```python
from build123d import *

# Parameters (mm, degrees)
BOSS_EXTRUDE1_DEPTH = 17
SKETCH2_W           = 17
SKETCH2_H           = 17
CUT_EXTRUDE1_DEPTH  = 13
SKETCH3_RX          = 4.47
SKETCH3_RY          = 3.075
CUT_EXTRUDE2_DEPTH  = 13
SKETCH5_RX          = 4.47
SKETCH5_RY          = 3.075
CUT_EXTRUDE3_DEPTH  = 13
SKETCH6_W           = 3.5
SKETCH6_H           = 1.5
BOSS_EXTRUDE2_DEPTH = 1
FILLET1_R           = 0.75
SKETCH7_W           = 1.5
SKETCH7_H           = 3.5
BOSS_EXTRUDE3_DEPTH = 1
FILLET2_R           = 0.75


with BuildPart() as part:
    # Sketch1 → Boss-Extrude1 (new body)
    with BuildSketch(Plane.XY):
        Polygon((0, 0), (0, 20), (3.029437252, 20), (20, 3.029437252), (20, 0), align=None)
    extrude(amount=BOSS_EXTRUDE1_DEPTH)

    # Sketch2 → Cut-Extrude1 (cut)
    with BuildSketch(Plane.XY.offset(2)):
        with Locations((11.5, 11.5)):
            Rectangle(SKETCH2_W, SKETCH2_H)
    extrude(amount=CUT_EXTRUDE1_DEPTH, mode=Mode.SUBTRACT)

    # Sketch3 → Cut-Extrude2 (cut)
    with BuildSketch(Plane(origin=(0, 0, 0), x_dir=(1, 0, 0), z_dir=(0, 1, 0))):
        with Locations((10.16, -8.425)):
            Ellipse(SKETCH3_RX, SKETCH3_RY)
    extrude(amount=CUT_EXTRUDE2_DEPTH, mode=Mode.SUBTRACT)

    # Sketch5 → Cut-Extrude3 (cut)
    with BuildSketch(Plane(origin=(0, 0, 0), x_dir=(0, 0, -1), z_dir=(1, 0, 0))):
        with Locations(Location((-8.375, 10.47), (0, 0, 90))):
            Ellipse(SKETCH5_RX, SKETCH5_RY)
    extrude(amount=CUT_EXTRUDE3_DEPTH, mode=Mode.SUBTRACT)

    # Sketch6 → Boss-Extrude2 (add)
    with BuildSketch(Plane(origin=(0, 0, 0), x_dir=(0, 0, -1), z_dir=(1, 0, 0))):
        with Locations((-8.25, 18.25)):
            Rectangle(SKETCH6_W, SKETCH6_H)
        with Locations((-8.25, 2.75)):
            Rectangle(SKETCH6_W, SKETCH6_H)
    extrude(amount=-BOSS_EXTRUDE2_DEPTH)

    # Fillet1
    fillet1_edges = [part.edges().sort_by_distance(p)[0] for p in [
        (-0.5, 2, 6.5),
        (-0.5, 17.5, 6.5),
        (-0.5, 2, 10),
        (-0.5, 3.5, 10),
        (-0.5, 3.5, 6.5),
        (-0.5, 17.5, 10),
        (-0.5, 19, 10),
        (-0.5, 19, 6.5),
    ]]
    fillet(fillet1_edges, radius=FILLET1_R - 0.0001)  # a hair under: the kernel refuses the full size

    # Sketch7 → Boss-Extrude3 (add)
    with BuildSketch(Plane(origin=(0, 0, 0), x_dir=(1, 0, 0), z_dir=(0, 1, 0))):
        with Locations((2.75, -8.25)):
            Rectangle(SKETCH7_W, SKETCH7_H)
        with Locations((18.25, -8.25)):
            Rectangle(SKETCH7_W, SKETCH7_H)
    extrude(amount=-BOSS_EXTRUDE3_DEPTH)

    # Fillet2
    fillet2_edges = [part.edges().sort_by_distance(p)[0] for p in [
        (3.5, -0.5, 6.5),
        (2, -0.5, 6.5),
        (2, -0.5, 10),
        (3.5, -0.5, 10),
        (17.5, -0.5, 10),
        (19, -0.5, 10),
        (17.5, -0.5, 6.5),
        (19, -0.5, 6.5),
    ]]
    fillet(fillet2_edges, radius=FILLET2_R - 0.0001)  # a hair under: the kernel refuses the full size


solid = part.part
```
Geometry: final body of the model. Coordinates: model frame, mm. A direction names the side the tool comes from. Round coordinates to 2 decimals unless told otherwise and drop trailing zeros. Write each loop counter-clockwise with the first axis right and the second up, starting at its lowest first coordinate (ties: lowest second). Pieces come first, ordered by that corner, then holes. Notation, with made-up numbers: (-39, -22) -> (-30, -22) arc R11 ccw to (-30, -18) -> close; hole circle Ø9 at (-40, 27). An arc over 180 degrees is marked (long way). Use CSV: the item, a comma, the result in double quotes. Start each with the question number.
Q1. Pull-direction query (Z, two-part tool) for faces 1 (the face through (9, 10, 2)), 2 (the face through (8, 8, 0)), 3 (the face through (19, -0.5, 8.3)); classes: pulls with the +Z half, pulls with the -Z half, needs draft (parallel to the pull), parting line crosses it, or undercut.
Q2. Section B-B (x = 16.25). Return loops of the section in (y, z), plus the area to 3 significant figures.
Q3. Section C-C (z = 8.75). Give the number of separate pieces and of enclosed holes in the cut face, plus the area to 3 significant figures.
Q4. First-contact query: pin 1 Ø3 at (y, z) = (14.5, 15) entering from +X; pin 2 Ø0.5 at (y, z) = (-0.5, 8.5) entering from +X; pin 3 Ø5 at (y, z) = (9.5, 7) entering from -X. Flat tips, straight axial feed; report the tip coordinate or a pass-through.
Q5. Line query: L1, parallel to Z at x = 13, y = 3.75; L2, parallel to X at y = 14.75, z = 4.75; L3, parallel to Y at x = 1, z = 8.5. Output: solid intervals per line, ascending.
Q6. Reachability of faces 4 (the face through (17.5, -0.5, 8.3)), 5 (the face through (-0.5, 19, 8.3)), 6 (the face through (-0.5, 17.5, 8.3)) from +Z, -Z, +X, -X, +Y, -Y: full face, straight path, thin tool, end or side. Return the list, or none.
Q7. Section D-D (x = 4.5). Return loops of the section in (y, z).
Q8. Section A-A (z = 12). Return loops of the section in (x, y), plus the area to 3 significant figures.
Result sheet:
1,face 1,"undercut"
1,face 2,"pulls with the -Z half"
1,face 3,"needs draft"
2,outline,"(0, 0) -> (6.78, 0) -> (6.78, 2) -> (3, 2) -> (3, 15) -> (6.78, 15) -> (6.78, 17) -> (0, 17) -> close"
2,area,"66.1 mm²"
3,separate pieces,"3"
3,enclosed holes,"0"
3,area,"63.7 mm²"
4,pin 1,"x = 10.03"
4,pin 2,"x = 19"
4,pin 3,"x = 0"
5,L1,"0 to 2, 15 to 17"
5,L2,"0 to 3"
5,L3,"0 to 6, 14.94 to 20"
6,face 4,"+Z, -Z, -Y"
6,face 5,"+Z, -Z, -X, +Y"
6,face 6,"+Z, -Z, -X"
7,outline,"(0, 0) -> (18.53, 0) -> (18.53, 2) -> (3, 2) -> (3, 15) -> (18.53, 15) -> (18.53, 17) -> (0, 17) -> close"
8,outline,"(0, 0) -> (20, 0) -> (20, 3) -> (3, 3) -> (3, 20) -> (0, 20) -> close"
8,area,"111 mm²"
